Check sheet for the modelled part. Datum: model origin and axes. Units: mm. A direction names the side the tool comes from. Coordinates: 2 decimals unless noted, no trailing zeros. Loops run counter-clockwise (first coordinate to the right, second up) from the corner with the lowest first, then second, coordinate; pieces in that order, holes last. Notation, with made-up numbers: M 17,46.5 L 75,46.5 A30 ccw 75,72.5 Z; hole C 42.5,74.5 d2. An arc over 180 degrees is marked long. Return JSON: item names as keys, results as strings.
from build123d import *

# Parameters (mm, degrees)
SKETCH1_R           = 10.71
SKETCH1_R_2         = 7.71
SKETCH1_W           = 10
SKETCH1_H           = 10
BOSS_EXTRUDE1_DEPTH = 16
SKETCH2_R           = 1.55
CUT_EXTRUDE1_DEPTH  = 34.263383725
SKETCH3_R           = 1.6
CUT_EXTRUDE2_DEPTH  = 34.074839332
CUT_EXTRUDE4_START  = -10
SKETCH4_W           = 5
SKETCH4_H           = 10
CUT_EXTRUDE4_DEPTH  = 10
FILLET1_R           = 3
BOSS_EXTRUDE2_DEPTH = 15
SKETCH10_R          = 13.75
SKETCH10_R_2        = 1.5
BOSS_EXTRUDE3_DEPTH = 10
FILLET2_R           = 2


with BuildPart() as part:
    # Sketch1 → Boss-Extrude1 (new body)
    # profile 1 of 2: a face of its own
    with BuildSketch(Plane(origin=(0, 0, 0), x_dir=(0, 0, -1), z_dir=(1, 0, 0))):
        Circle(SKETCH1_R)
        Circle(SKETCH1_R_2, mode=Mode.SUBTRACT)
    # profile 2 of 2: a face of its own
    with BuildSketch(Plane(origin=(0, 0, 0), x_dir=(0, 0, -1), z_dir=(1, 0, 0))):
        with Locations((0, 14.471224842)):
            Rectangle(SKETCH1_W, SKETCH1_H)
    extrude(amount=BOSS_EXTRUDE1_DEPTH)

    # Sketch2 → Cut-Extrude1 (cut, through all)
    with BuildSketch(Plane(origin=(16, 0, 11), x_dir=(0, 0, 1), z_dir=(-1, 0, 0))):
        with Locations((-11, 14.471224842)):
            Circle(SKETCH2_R)
    extrude(amount=CUT_EXTRUDE1_DEPTH, mode=Mode.SUBTRACT)

    # Sketch3 → Cut-Extrude2 (cut, through all)
    with BuildSketch(Plane.XY.offset(10.71)):
        with Locations((8, 0)):
            Circle(SKETCH3_R)
    extrude(amount=-CUT_EXTRUDE2_DEPTH, mode=Mode.SUBTRACT)

    # Sketch4 → Cut-Extrude4 (cut)
    with BuildSketch(Plane(origin=(0, 19.471224842, 0), x_dir=(1, 0, 0), z_dir=(0, 1, 0)).offset(CUT_EXTRUDE4_START)):
        with Locations((2.5, 0)):
            Rectangle(SKETCH4_W, SKETCH4_H)
        with Locations((13.5, 0)):
            Rectangle(SKETCH4_W, SKETCH4_H)
    extrude(amount=CUT_EXTRUDE4_DEPTH, mode=Mode.SUBTRACT)

    # Fillet1
    fillet1_edges = [part.edges().sort_by_distance(p)[0] for p in [
        (8, 19.471224842, 5),
        (8, 19.471224842, -5),
    ]]
    fillet(fillet1_edges, radius=FILLET1_R)

    # Sketch8 → Boss-Extrude2 (add)
    with BuildSketch(Plane(origin=(16, 0, 0), x_dir=(0, 0, -1), z_dir=(1, 0, 0))):
        with BuildLine():
            Line((5, 9.471224842), (-5, 9.471224842))
            ThreePointArc((-5, 9.471224842), (0, -10.71), (5, 9.471224842))
        make_face()
    extrude(amount=BOSS_EXTRUDE2_DEPTH)

    # Sketch10 → Boss-Extrude3 (add)
    with BuildSketch(Plane(origin=(31, 0, 0), x_dir=(0, 0, -1), z_dir=(1, 0, 0))):
        Circle(SKETCH10_R)
        Circle(SKETCH10_R_2, mode=Mode.SUBTRACT)
    extrude(amount=-BOSS_EXTRUDE3_DEPTH)

    # Fillet2
    fillet2_edges = [part.edges().sort_by_distance(p)[0] for p in [
        (31, 0, 13.75),
        (21, 0, 13.75),
    ]]
    fillet(fillet2_edges, radius=FILLET2_R)


solid = part.part
1) Section check C-C on x = 28. Record the cut outline in (y, z), then the cut area to 3 significant figures.
Answers:
{"outline": "C 0,0 d27.5", "area": "594 mm²"}
2) Section check B-B on x = 8. Record the cut outline in (y, z).
Answers:
{"outline": "M -1.6,-10.59 L -1.6,-7.54 A7.71 cw -1.6,7.54 L -1.6,10.59 A10.71 ccw Z; M 1.6,-10.59 A10.71 ccw 9.47,-5 L 16.47,-5 A3 ccw 19.47,-2 L 19.47,2 A3 ccw 16.47,5 L 9.47,5 A10.71 ccw 1.6,10.59 L 1.6,7.54 A7.71 cw 1.6,-7.54 Z; hole C 14.47,0 d3.1"}
3) Section check A-A on y = 0. Record the cut outline in (x, z), then the cut area to 3 significant figures.
Answers:
{"outline": "M 0,-10.71 L 6.4,-10.71 L 6.4,-7.71 L 0,-7.71 Z; M 0,7.71 L 6.4,7.71 L 6.4,10.71 L 0,10.71 Z; M 9.6,-10.71 L 21,-10.71 L 21,-11.75 A2 ccw 23,-13.75 L 29,-13.75 A2 ccw 31,-11.75 L 31,11.75 A2 ccw 29,13.75 L 23,13.75 A2 ccw 21,11.75 L 21,10.71 L 9.6,10.71 L 9.6,7.71 L 16,7.71 L 16,-7.71 L 9.6,-7.71 Z", "area": "455 mm²"}
4) Go/stop test with flat-tipped pins: pin 1 Ø3 at (x, z) = (15.5, -1) entering from +Y; pin 2 Ø3 at (y, z) = (14.47, 0) entering from -X; pin 3 Ø3 at (x, y) = (9, 12.5) entering from +Z; pin 4 Ø2.5 at (x, y) = (8, 0) entering from -Z. Record where each tip stops, or that it passes through.
Answers:
{"pin 1": "y = 9.47", "pin 2": "x = 21.42", "pin 3": "z = 5", "pin 4": "through"}
5) Scan lines: line 1 along Y through (x, z) = (5.25, 0); line 2 along X through (y, z) = (0, -9.25); line 3 along Z through (x, y) = (4.75, 0). Record each from-to range of solid material in increasing order. Write a range as [from, to].
Answers:
{"line 1": "[-10.71, -7.71], [7.71, 12.92], [16.02, 19.47]", "line 2": "[0, 6.4], [9.6, 31]", "line 3": "[-10.71, -7.71], [7.71, 10.71]"}
6) Set-up check for faces 5 (the face through (2, 9.471, 0)), 6 (the face through (21, 10, 0)), 7 (the face through (8, 13, -5)), 8 (the face through (8.04, 12.96, -0.34)): record each of +Z, -Z, +X, -X, +Y, -Y from which the full face is reachable in a straight line by a thin tool's end or side.
Answers:
{"face 5": "+Z, -Z, -X, +Y", "face 6": "none", "face 7": "-Z, -X, +Y", "face 8": "-X"}
7) Section check D-D on x = 13.5. Record the cut outline in (y, z).
Answers:
{"outline": "M 9.47,-5 L 9.47,5 A10.71 ccw long Z; hole C 0,0 d15.42"}
8) Draft check along Y on faces 1 (the face through (6.4, 0.07, 9.15)), 2 (the face through (16, 0, 0)), 3 (the face through (5, 13, 1)), 4 (the face through (8.042, 18.616, -4.098)). Enter one of: +Y half, -Y half, draft (parallel to the pull), parting line (faces both ways), or undercut.
Answers:
{"face 1": "undercut", "face 2": "undercut", "face 3": "draft", "face 4": "+Y half"}
